from build123d import *

# Parameters (mm, degrees)
AUFSATZ_LINEAR_AUSTRAGEN1_DEPTH = 6
AUFSATZ_LINEAR_START            = 6
AUFSATZ_LINEAR_AUSTRAGEN4_DEPTH = 2
AUFSATZ_LINEAR_START_2          = -6
AUFSATZ_LINEAR_AUSTRAGEN5_DEPTH = 2
SKIZZE2_R                       = 1.5
SCHNITT_LINEAR_AUSTRAGEN1_DEPTH = 4


with BuildPart() as part:
    # Skizze1 → Aufsatz-Linear austragen1 (new body, symmetric)
    with BuildSketch(Plane(origin=(0, 0, 0), x_dir=(0, 0, -1), z_dir=(1, 0, 0))):
        Polygon((0, 20), (0, 0), (-20, 0), (-20, 3), (-3, 3), (-3, 20), align=None)
    extrude(amount=AUFSATZ_LINEAR_AUSTRAGEN1_DEPTH, both=True)

    # Skizze1_3 → Aufsatz-Linear austragen4 (add)
    with BuildSketch(Plane(origin=(0, 0, 0), x_dir=(0, 0, -1), z_dir=(1, 0, 0)).offset(AUFSATZ_LINEAR_START)):
        Polygon((-3, 3), (-3, 20), (-20, 3), align=None)
    extrude(amount=-AUFSATZ_LINEAR_AUSTRAGEN4_DEPTH)

    # Skizze1_4 → Aufsatz-Linear austragen5 (add)
    with BuildSketch(Plane(origin=(0, 0, 0), x_dir=(0, 0, -1), z_dir=(1, 0, 0)).offset(AUFSATZ_LINEAR_START_2)):
        Polygon((-3, 3), (-3, 20), (-20, 3), align=None)
    extrude(amount=AUFSATZ_LINEAR_AUSTRAGEN5_DEPTH)

    # Skizze2 → Schnitt-Linear austragen1 (cut, through all)
    with BuildSketch(Plane.XY.offset(3)):
        with Locations((0, 11.5)):
            Circle(SKIZZE2_R)
    schnitt_linear_austragen1 = extrude(amount=-SCHNITT_LINEAR_AUSTRAGEN1_DEPTH, mode=Mode.SUBTRACT)

    # Spiegeln2: Schnitt-Linear austragen1 across plane
    add(schnitt_linear_austragen1.mirror(Plane(origin=(0, 0, 0), x_dir=(0, 0.707106781, 0.707106781), z_dir=(0, -0.707106781, 0.707106781))), mode=Mode.SUBTRACT)


solid = part.part
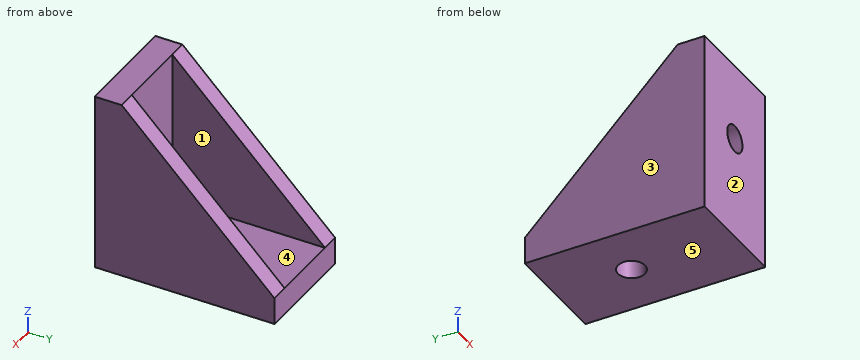
Work out the finished part from the listing and answer in its coordinate system (mm). Face numbers are marked on the shaded views. A direction names the side the tool comes from. Give positions to 0.01 mm unless a question says otherwise; leave off trailing zeros. Loops run counter-clockwise (first coordinate to the right, second up) from the corner with the lowest first, then second, coordinate; pieces in that order, holes last. Notation, with made-up numbers: (33.5, 87.5) -> (49.5, 87.5) arc R24 cw to (49.5, 106.5) -> close; hole circle Ø4 at (35.25, -11). An arc over 180 degrees is marked (long way). Use a Markdown table: item, result. Add a question column.
1. Section A-A on z = 11.5 is taken. Determine the outline of the cut face in (x, y).
2. Section D-D on y = 7.25 is taken. Determine the outline of the cut face in (x, z).
3. Find the intervals of material crossed by probe 1 along Y at (x, z) = (0, 1.6); probe 2 along X at (y, z) = (3.25, 12.25), in increasing order.
4. Flat-ended cylindrical pins translate along their axes: pin 1 Ø1.5 at (x, y) = (0, 17.5) entering from +Z; pin 2 Ø4 at (x, z) = (-1, 12) entering from +Y; pin 3 Ø1.5 at (x, z) = (3.5, 12) entering from +Y. Find the tip coordinate at first contact, or state that the pin passes through.
5. Section B-B on x = 0 is taken. Determine the outline of the cut face in (y, z).
6. Determine the mould class of the marked faces 1, 2 and 3 for opening direction X: released by +X, released by -X, zero draft, split by the parting line, or undercut.
7. Section C-C on y = 2.25 is taken. Determine the outline of the cut face in (x, z).
8. For the marked faces 4 and 5, determine the directions among +Z, -Z, +X, -X, +Y, -Y from which every point of the face is accessible in a straight line to the end or side of a thin tool.
Results below:
| question | item | result |
|---|---|---|
| 1 | outline | (-6, 0) -> (-1.5, 0) -> (-1.5, 3) -> (-4, 3) -> (-4, 11.5) -> (-6, 11.5) -> close; (1.5, 0) -> (6, 0) -> (6, 11.5) -> (4, 11.5) -> (4, 3) -> (1.5, 3) -> close |
| 2 | outline | (-6, 0) -> (6, 0) -> (6, 15.75) -> (4, 15.75) -> (4, 3) -> (-4, 3) -> (-4, 15.75) -> (-6, 15.75) -> close |
| 3 | probe 1 | y = 0 to 10, 13 to 20 |
| 3 | probe 2 | x = -6 to -4, 4 to 6 |
| 4 | pin 1 | stops at z = 3 |
| 4 | pin 2 | stops at y = 3 |
| 4 | pin 3 | stops at y = 11.56 |
| 5 | outline | (0, 0) -> (10, 0) -> (10, 3) -> (3, 3) -> (3, 10) -> (0, 10) -> close; (0, 13) -> (3, 13) -> (3, 20) -> (0, 20) -> close; (13, 0) -> (20, 0) -> (20, 3) -> (13, 3) -> close |
| 6 | face 1 | undercut |
| 6 | face 2 | zero draft |
| 6 | face 3 | released by -X |
| 7 | outline | (-6, 0) -> (6, 0) -> (6, 20) -> (-6, 20) -> close; hole circle Ø3 at (0, 11.5) |
| 8 | face 4 | +Z, +Y |
| 8 | face 5 | -Z, +X, -X, +Y, -Y |
